Part model, mm, in its own coordinate system. A direction names the side the tool comes from. Give positions to 0.01 mm unless a question says otherwise; leave off trailing zeros. Order: outer loops, then holes, each group sorted by start corner. A loop starts at its lowest first (then second) coordinate and runs counter-clockwise, first axis right, second up. Notation, with made-up numbers: (56.25, 19) -> (63.25, 19) arc R19 cw to (63.25, 37) -> close; hole circle Ø11 at (44, 66). An arc over 180 degrees is marked (long way). Write item = value, one per line. Start each with the question number.
Item 1: Band-saw the part on B-B on z = 0. Write the cut outline in (x, y), plus the area to 3 significant figures.
Item 2: Drill centre lines: line 1 along X through (y, z) = (-2.5, 47.5); line 2 along Y through (x, z) = (29, 27); line 3 along X through (y, z) = (1.25, 26). Where is each one in solid material? Low to high.
Item 3: Band-saw the part on D-D on x = 8. Write the cut outline in (y, z), plus the area to 3 significant figures.
Item 4: Band-saw the part on A-A on y = -3.25. Write the cut outline in (x, z).
Item 5: Band-saw the part on C-C on x = 0. Write the cut outline in (y, z).
Item 6: Pull direction X, two halves, no side cores. Call faces 1 (the face through (-4.776, -1.549, -9.857)), 2 (the face through (-5.775, -1.549, 46.222)), 3 (the face through (-8.83, 1, 19)), 4 (the face through (45.4, 0, -8.3)): +X half, -X half, draft (parallel to the pull), parting line (faces both ways), or undercut.
Item 7: Tool access for faces 5 (the face through (43, 1, 44.471)), 6 (the face through (37.054, 0.986, 0.672)), 7 (the face through (45.4, 0, 49.7)), 8 (the face through (-8, 0, 50)): list every direction of +Z, -Z, +X, -X, +Y, -Y with a clear straight run to the whole face (end or side of a thin tool).
Item 8: Flat gauge pins, fed straight in: P1, Ø2, axis at x = 19, z = 14, coming from the -Y side; P2, Ø0.9, axis at x = -6.5, z = -11.5, coming from the -Y side; P3, Ø0.6, axis at y = 1, z = 17.5, coming from the +X side. Where does each tip first touch, or does it go through?
```python
from build123d import *

# Parameters (mm, degrees)
SKETCH2_W           = 55
SKETCH2_H           = 64
SKETCH2_R           = 1.25
SKETCH2_R_2         = 1.249934
BOSS_EXTRUDE1_DEPTH = 2
SKETCH4_W           = 7
SKETCH4_H           = 52
CUT_EXTRUDE1_DEPTH  = 2
FILLET1_R           = 1
BOSS_EXTRUDE2_START = -7
SKETCH5_R           = 3
SKETCH5_R_2         = 1.25
BOSS_EXTRUDE2_DEPTH = 7


with BuildPart() as part:
    # Sketch2 → Boss-Extrude1 (new body)
    with BuildSketch(Plane(origin=(0, 0, 0), x_dir=(1, 0, 0), z_dir=(0, 1, 0))):
        with Locations((18.669829868, -18.471180694)):
            Rectangle(SKETCH2_W, SKETCH2_H)
        with Locations(Location((-5.830170132, 10.528819306, 0), (0, 0, 270))):
            Circle(SKETCH2_R, mode=Mode.SUBTRACT)
        with Locations(Location((-5.830170132, -47.471180694, 0), (0, 0, 270))):
            Circle(SKETCH2_R, mode=Mode.SUBTRACT)
        with Locations(Location((43.169829868, -47.471180694, 0), (0, 0, 270))):
            Circle(SKETCH2_R, mode=Mode.SUBTRACT)
        with Locations(Location((43.169829868, 10.528819306, 0), (0, 0, 270))):
            Circle(SKETCH2_R, mode=Mode.SUBTRACT)
        with Locations(Location((0, 0, 0), (0, 0, 270))):
            Circle(SKETCH2_R_2, mode=Mode.SUBTRACT)
        with Locations(Location((35.999928, 0, 0), (0, 0, 270))):
            Circle(SKETCH2_R_2, mode=Mode.SUBTRACT)
        with Locations(Location((0, -35.999928, 0), (0, 0, 270))):
            Circle(SKETCH2_R_2, mode=Mode.SUBTRACT)
        with Locations(Location((35.999928, -35.999928, 0), (0, 0, 270))):
            Circle(SKETCH2_R_2, mode=Mode.SUBTRACT)
    extrude(amount=BOSS_EXTRUDE1_DEPTH)

    # Sketch4 → Cut-Extrude1 (cut)
    with BuildSketch(Plane(origin=(0, 2, 0), x_dir=(1, 0, 0), z_dir=(0, 1, 0))):
        with Locations((42.669829868, -18.471180694)):
            Rectangle(SKETCH4_W, SKETCH4_H)
    extrude(amount=-CUT_EXTRUDE1_DEPTH, mode=Mode.SUBTRACT)

    # Fillet1
    fillet1_edges = [part.edges().sort_by_distance(p)[0] for p in [
        (46.169829868, 1, -13.528819306),
        (46.169829868, 1, 50.471180694),
        (-8.830170132, 1, 50.471180694),
        (-8.830170132, 1, -13.528819306),
        (46.169829868, 1, -7.528819306),
        (46.169829868, 1, 44.471180694),
        (39.169829868, 1, 44.471180694),
        (39.169829868, 1, -7.528819306),
    ]]
    fillet(fillet1_edges, radius=FILLET1_R)

    # Sketch5 → Boss-Extrude2 (add)
    # profile 1 of 4: a face of its own
    with BuildSketch(Plane(origin=(0, 2, 0), x_dir=(1, 0, 0), z_dir=(0, 1, 0)).offset(BOSS_EXTRUDE2_START)):
        with Locations(Location((-5.830170132, 10.528819306, 0), (0, 0, 270))):
            Circle(SKETCH5_R)
        with Locations(Location((-5.830170132, 10.528819306, 0), (0, 0, 270))):
            Circle(SKETCH5_R_2, mode=Mode.SUBTRACT)
    # profile 2 of 4: a face of its own
    with BuildSketch(Plane(origin=(0, 2, 0), x_dir=(1, 0, 0), z_dir=(0, 1, 0)).offset(BOSS_EXTRUDE2_START)):
        with Locations(Location((43.169829868, 10.528819306, 0), (0, 0, 270))):
            Circle(SKETCH5_R)
        with Locations(Location((43.169829868, 10.528819306, 0), (0, 0, 270))):
            Circle(SKETCH5_R_2, mode=Mode.SUBTRACT)
    # profile 3 of 4: a face of its own
    with BuildSketch(Plane(origin=(0, 2, 0), x_dir=(1, 0, 0), z_dir=(0, 1, 0)).offset(BOSS_EXTRUDE2_START)):
        with Locations(Location((43.169829868, -47.471180694, 0), (0, 0, 270))):
            Circle(SKETCH5_R)
        with Locations(Location((43.169829868, -47.471180694, 0), (0, 0, 270))):
            Circle(SKETCH5_R_2, mode=Mode.SUBTRACT)
    # profile 4 of 4: a face of its own
    with BuildSketch(Plane(origin=(0, 2, 0), x_dir=(1, 0, 0), z_dir=(0, 1, 0)).offset(BOSS_EXTRUDE2_START)):
        with Locations(Location((-5.830170132, -47.471180694, 0), (0, 0, 270))):
            Circle(SKETCH5_R)
        with Locations(Location((-5.830170132, -47.471180694, 0), (0, 0, 270))):
            Circle(SKETCH5_R_2, mode=Mode.SUBTRACT)
    extrude(amount=BOSS_EXTRUDE2_DEPTH)


solid = part.part
```
Values found:
q1.outline = (-8.83, 0) -> (-1.25, 0) -> (-1.25, 2) -> (-8.83, 2) -> close; (1.25, 0) -> (34.75, 0) -> (34.75, 2) -> (1.25, 2) -> close; (37.25, 0) -> (39.17, 0) -> (39.17, 2) -> (37.25, 2) -> close
q1.area = 86.0 mm^2
q2.line_1 = -8.83 to -7.08, -4.58 to -2.83, 40.17 to 41.92, 44.42 to 46.17
q2.line_2 = 0 to 2
q2.line_3 = -8.83 to 39.17
q3.outline = (0, -13.53) -> (2, -13.53) -> (2, 50.47) -> (0, 50.47) -> close
q3.area = 128 mm^2
q4.outline = circle Ø6 at (-5.83, -10.53); circle Ø6 at (-5.83, 47.47); circle Ø6 at (43.17, -10.53); circle Ø6 at (43.17, 47.47); hole circle Ø2.5 at (-5.83, -10.53); hole circle Ø2.5 at (-5.83, 47.47); hole circle Ø2.5 at (43.17, -10.53); hole circle Ø2.5 at (43.17, 47.47)
q5.outline = (0, -13.53) -> (2, -13.53) -> (2, -1.25) -> (0, -1.25) -> close; (0, 1.25) -> (2, 1.25) -> (2, 34.75) -> (0, 34.75) -> close; (0, 37.25) -> (2, 37.25) -> (2, 50.47) -> (0, 50.47) -> close
q6.face_1 = undercut
q6.face_2 = undercut
q6.face_3 = -X half
q6.face_4 = draft
q7.face_5 = +X, +Y, -Y
q7.face_6 = +Y, -Y
q7.face_7 = +Z, +X, -Y
q7.face_8 = +Z, -X, -Y
q8.P1 = 0
q8.P2 = -5
q8.P3 = 39.17
